Here's how the part is built. I have some questions about the finished solid (model axes, mm). Face numbers are marked on the shaded views. Give positions to 0.01 mm unless a question says otherwise; leave off trailing zeros. Write each loop counter-clockwise with the first axis right and the second up, starting at its lowest first coordinate (ties: lowest second). Pieces come first, ordered by that corner, then holes. Notation, with made-up numbers: (-25.75, 74) - (-21.75, 74) arc R17 ccw to (-21.75, 79) - close; hole circle Ø3 at (26.5, 57). An arc over 180 degrees is marked (long way). Use one line per item in the form item = value. Start each with the question number.
from build123d import *

# Parameters (mm, degrees)
SKETCH1_W           = 36
SKETCH1_H           = 27
BOSS_EXTRUDE1_DEPTH = 7
CUT_EXTRUDE1_DEPTH  = 0.2
BOSS_EXTRUDE2_DEPTH = 0.2
BOSS_EXTRUDE3_DEPTH = 0.2


with BuildPart() as part:
    # Sketch1 → Boss-Extrude1 (new body)
    with BuildSketch(Plane.XY):
        Rectangle(SKETCH1_W, SKETCH1_H)
    extrude(amount=BOSS_EXTRUDE1_DEPTH)

    # Sketch2 → Cut-Extrude1 (cut)
    with BuildSketch(Plane.XY.offset(7)):
        with BuildLine():
            Line((-9.9, -9), (9.9, -9))
            ThreePointArc((9.9, -9), (11.03137085, -8.53137085), (11.5, -7.4))
            Line((11.5, -7.4), (11.5, 7.4))
            ThreePointArc((11.5, 7.4), (11.03137085, 8.53137085), (9.9, 9))
            Line((9.9, 9), (-9.9, 9))
            ThreePointArc((-9.9, 9), (-11.03137085, 8.53137085), (-11.5, 7.4))
            Line((-11.5, 7.4), (-11.5, -7.4))
            ThreePointArc((-11.5, -7.4), (-11.03137085, -8.53137085), (-9.9, -9))
        make_face()
    extrude(amount=-CUT_EXTRUDE1_DEPTH, mode=Mode.SUBTRACT)

    # Sketch3 → Boss-Extrude2 (add)
    with BuildSketch(Plane.XY.offset(6.8)):
        with BuildLine():
            Line((2.9, 7.5), (3.461670446, 2.49974195))
            ThreePointArc((3.461670446, 2.49974195), (3.767203859, 2.093615319), (4.270423503, 2.164745466))
            Line((4.270423503, 2.164745466), (8.203300859, 5.303300859))
            Line((8.203300859, 5.303300859), (5.064745466, 1.370423503))
            ThreePointArc((5.064745466, 1.370423503), (4.993615319, 0.867203859), (5.39974195, 0.561670446))
            Line((5.39974195, 0.561670446), (10.4, 0))
            Line((10.4, 0), (5.39974195, -0.561670446))
            ThreePointArc((5.39974195, -0.561670446), (4.993615319, -0.867203859), (5.064745466, -1.370423503))
            Line((5.064745466, -1.370423503), (8.203300859, -5.303300859))
            Line((8.203300859, -5.303300859), (4.270423503, -2.164745466))
            ThreePointArc((4.270423503, -2.164745466), (3.767203859, -2.093615319), (3.461670446, -2.49974195))
            Line((3.461670446, -2.49974195), (2.9, -7.5))
            Line((2.9, -7.5), (2.338329554, -2.49974195))
            ThreePointArc((2.338329554, -2.49974195), (2.032796141, -2.093615319), (1.529576497, -2.164745466))
            Line((1.529576497, -2.164745466), (-2.403300859, -5.303300859))
            Line((-2.403300859, -5.303300859), (0.735254534, -1.370423503))
            ThreePointArc((0.735254534, -1.370423503), (0.806384681, -0.867203859), (0.40025805, -0.561670446))
            Line((0.40025805, -0.561670446), (-4.6, 0))
            Line((-4.6, 0), (0.40025805, 0.561670446))
            ThreePointArc((0.40025805, 0.561670446), (0.806384681, 0.867203859), (0.735254534, 1.370423503))
            Line((0.735254534, 1.370423503), (-2.403300859, 5.303300859))
            Line((-2.403300859, 5.303300859), (1.529576497, 2.164745466))
            ThreePointArc((1.529576497, 2.164745466), (2.032796141, 2.093615319), (2.338329554, 2.49974195))
            Line((2.338329554, 2.49974195), (2.9, 7.5))
        make_face()
    extrude(amount=BOSS_EXTRUDE2_DEPTH)

    # Sketch5 → Boss-Extrude3 (add)
    with BuildSketch(Plane.XY.offset(6.8)):
        Polygon((-5.413360388, 2.785130003), (-4.913360388, 1.785130003), (-5.413360388, 0.785130003), (-5.913360388, 1.785130003), align=None)
        Polygon((8.513360388, 3.325130003), (9.013360388, 2.325130003), (8.513360388, 1.325130003), (8.013360388, 2.325130003), align=None)
        Polygon((4.725130003, 5.613360388), (5.225130003, 6.613360388), (5.725130003, 5.613360388), (5.225130003, 4.613360388), align=None)
        Polygon((0.574869997, 6.613360388), (1.074869997, 5.613360388), (0.574869997, 4.613360388), (0.074869997, 5.613360388), align=None)
        Polygon((-2.713360388, 3.325130003), (-2.213360388, 2.325130003), (-2.713360388, 1.325130003), (-3.213360388, 2.325130003), align=None)
        Polygon((-7.213360388, 1.135887753), (-6.713360388, 0.135887753), (-7.213360388, -0.864112247), (-7.713360388, 0.135887753), align=None)
        Polygon((-9.808959232, 1), (-9.308959232, 0), (-9.808959232, -1), (-10.308959232, 0), align=None)
    extrude(amount=BOSS_EXTRUDE3_DEPTH)


solid = part.part
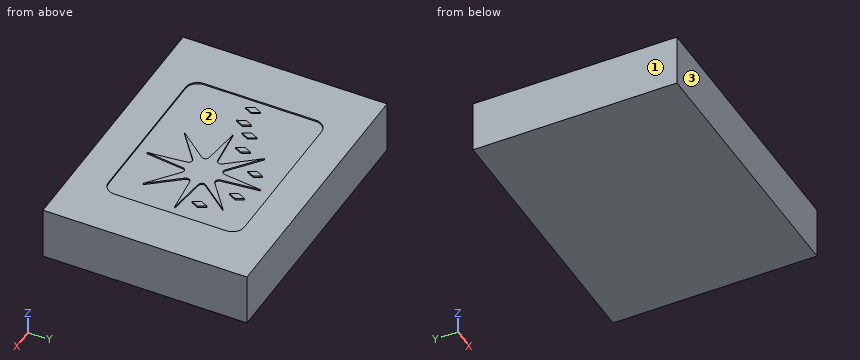
1. Please list where this line runs through material, in increasing order: line 1 (Z direction, x = -1, y = 8.75).
2. We'd pull the mould along X, two halves only. Please class the marked faces 1, 2 and 3: pulls with the +X half, pulls with the -X half, needs draft (parallel to the pull), parting line crosses it, or undercut.
3. I want a section at B-B, the plane y = 3.75. List the corners of the cut face in (x, z) for me, then the cut area to 3 significant figures.
4. For P1, Ø1.5, axis at x = 6.5, y = 8, coming from the +Z side, with a flat end and sliding along its axis, tell me the tip position at first contact or that it passes through.
5. I want a section at A-A, the plane x = 7. List the corners of the cut face in (y, z) for me.
Result sheet:
q1.line_1 = 0 to 6.8
q2.face_1 = pulls with the -X half
q2.face_2 = undercut
q2.face_3 = needs draft
q3.outline = (-18, 0) - (18, 0) - (18, 7) - (11.5, 7) - (11.5, 6.8) - (6.96, 6.8) - (6.96, 7) - (6.26, 7) - (6.26, 6.8) - (3.32, 6.8) - (3.32, 7) - (2.48, 7) - (2.48, 6.8) - (-0.46, 6.8) - (-0.46, 7) - (-1.16, 7) - (-1.16, 6.8) - (-11.5, 6.8) - (-11.5, 7) - (-18, 7) - close
q3.area = 248 mm2
q4.P1 = 6.8
q5.outline = (-13.5, 0) - (13.5, 0) - (13.5, 7) - (9, 7) - (9, 6.8) - (4.34, 6.8) - (4.34, 7) - (3.8, 7) - (3.8, 6.8) - (0.38, 6.8) - (0.38, 7) - (-0.38, 7) - (-0.38, 6.8) - (-3.8, 6.8) - (-3.8, 7) - (-4.34, 7) - (-4.34, 6.8) - (-9, 6.8) - (-9, 7) - (-13.5, 7) - close
